Source: CAD feature listing. Evaluate the final solid. Frame: model axes, mm. A direction names the side the tool comes from. Coordinates: 2 decimals unless noted, no trailing zeros. Order: outer loops, then holes, each group sorted by start corner. A loop starts at its lowest first (then second) coordinate and runs counter-clockwise, first axis right, second up. Notation, with made-up numbers: (4.25, 51.25) -> (13.25, 51.25) arc R29 ccw to (13.25, 86.25) -> close; hole circle Ø3 at (15, -36.5). An arc over 180 degrees is marked (long way). Write item = value, one per line. Start each with the question number.
Item 1: Section query B-B (x = -144). Output: boundary loops of the cut face in (y, z).
Item 2: Ray query, line 1 along Z through (x, y) = (-213, -80); line 2 along X through (y, z) = (55, 34); line 3 along Y through (x, z) = (-111, 0). Return the intervals inside material, ascending. Write a range as [from, to].
Item 3: Mould query, pull axis X, two halves, no side actions, for faces 1 (the cylindrical face through (-129.529, -15.77, -50.076)), 2 (the flat face through (-95, -28, 0)), 3 (the cylindrical face through (-215.14, -80.33, -72.507)), 4 (the flat face through (-77.5, 22.3, -12.1)). Classes: released by +X, released by -X, zero draft, split by the parting line, or undercut.
Item 4: Set-up query: faces 5 (the flat face through (-215, -1, -105)), 6 (the cylindrical face through (-215.14, 75.436, 74.048)), 7 (the flat face through (-215, 105, -1)), 8 (the cylindrical face through (-9.86, 93.676, 1.139)), 9 (the flat face through (-205, 48, -48)). Return all of +Z, -Z, +X, -X, +Y, -Y with unobstructed straight access to the full face (end or side cutting, diameter ignored); none if empty.
Item 5: Section query D-D (y = -65.5). Output: boundary loops of the cut face in (x, z), then the cut area to 3 significant figures.
Item 6: Section query A-A (y = 97.5). Output: boundary loops of the cut face in (x, z), then the cut area to 3 significant figures.
Item 7: Section query C-C (z = 0). Count the separate pieces of the cut face and the enclosed holes in it, then the cut area to 3 significant figures.
Item 8: Contact query for flat-ended pins moving along their axis: pin 1 (6 mm diameter, centred on x = -219, y = 38, fed in from -Z); pin 2 (5 mm diameter, centred on x = -149, y = 18.5, fed in from +Z); pin 3 (6 mm diameter, centred on x = -114, y = 49.5, fed in from -Z); pin 4 (5 mm diameter, centred on x = -200.5, y = -76.5, fed in from +Z). Output: stop coordinate, or through.
```python
from build123d import *

# Parameters (mm, degrees)
CUT_EXTRUDE_1_REACH      = 275.542
SKETCH_2_R               = 8.75
PATTERN_CIRCULAR_1_COUNT = 4
SKETCH_3_W               = 210
SKETCH_3_H               = 210
SKETCH_3_R               = 28.7125
EXTRUDE_1_DEPTH          = 20
SKETCH_4_R               = 7.5
CUT_EXTRUDE_2_DEPTH      = 20
FILLET_1_R               = 22
PATTERN_CIRCULAR_5_COUNT = 4
FILLET_2_R               = 3
SKETCH_5_R               = 28.7125
SKETCH_5_R_2             = 27.5
EXTRUDE_2_DEPTH          = 17.5
FILLET_3_R               = 3


with BuildPart() as part:
    # Эскиз1 → Повернуть1 (revolve)
    with BuildSketch(Plane.XY, mode=Mode.PRIVATE) as revolve_1_sk:
        Polygon((0, 37.5), (0, 110), (-20, 110), (-20, 60), (-55, 52.5), (-205, 52.5), (-205, 105), (-225, 105), (-225, 62.5), (-210, 62.5), (-210, 28.7125), (-160, 28.7125), (-160, 40), (-95, 40), (-95, 28.7125), (-77.5, 28.7125), (-77.5, 25), align=None)
    revolve(revolve_1_sk.sketch.rotate(Axis((0, 0, 0), (-1, 0, 0)), 90), axis=Axis((0, 0, 0), (-1, 0, 0)))

    # Эскиз2 → Вырез-Вытянуть1 (cut, up to next)
    with BuildSketch(Plane(origin=(0, 0, 0), x_dir=(0, 0, -1), z_dir=(1, 0, 0)), mode=Mode.PRIVATE) as cut_extrude_1_sk1:
        with Locations((0, 85)):
            Circle(SKETCH_2_R)
    cut_extrude_1_tool1 = extrude(cut_extrude_1_sk1.sketch, amount=-CUT_EXTRUDE_1_REACH, mode=Mode.PRIVATE) & part.part
    cut_extrude_1 = cut_extrude_1_tool1.solids().sort_by_distance((0, 85, 0))[0]
    add(cut_extrude_1, mode=Mode.SUBTRACT)

    # Круговой массив1: Вырез-Вытянуть1 ×4 about axis
    pattern_circular_1_axis = Axis((0, 0, 0), (1, 0, 0))
    for i in range(1, PATTERN_CIRCULAR_1_COUNT):
        add(cut_extrude_1.rotate(pattern_circular_1_axis, i * 360 / PATTERN_CIRCULAR_1_COUNT), mode=Mode.SUBTRACT)

    # Эскиз3 → Бобышка-Вытянуть1 (add)
    with BuildSketch(Plane.ZY.offset(225)):
        Rectangle(SKETCH_3_W, SKETCH_3_H)
        with Locations(Location((0, 0, 0), (0, 0, 180))):
            Circle(SKETCH_3_R, mode=Mode.SUBTRACT)
    extrude(amount=-EXTRUDE_1_DEPTH)

    # Эскиз4 → Вырез-Вытянуть2 (cut)
    with BuildSketch(Plane.ZY.offset(225)):
        with Locations((80, 80)):
            Circle(SKETCH_4_R)
    cut_extrude_2 = extrude(amount=-CUT_EXTRUDE_2_DEPTH, mode=Mode.SUBTRACT)

    # Скругление1
    fillet_1_edges = [part.edges().sort_by_distance(p)[0] for p in [
        (-215, 105, 105),
        (-215, -105, 105),
        (-215, -105, -105),
        (-215, 105, -105),
    ]]
    fillet(fillet_1_edges, radius=FILLET_1_R)

    # Круговой массив5: Вырез-Вытянуть2 ×4 about axis
    pattern_circular_5_axis = Axis((0, 0, 0), (1, 0, 0))
    for i in range(1, PATTERN_CIRCULAR_5_COUNT):
        add(cut_extrude_2.rotate(pattern_circular_5_axis, i * 360 / PATTERN_CIRCULAR_5_COUNT), mode=Mode.SUBTRACT)

    # Скругление2
    fillet_2_edges = [part.edges().sort_by_distance(p)[0] for p in [
        (-160, 0, 40),
        (-95, 0, 40),
    ]]
    fillet(fillet_2_edges, radius=FILLET_2_R)

    # Эскиз5 → Бобышка-Вытянуть2 (add)
    with BuildSketch(Plane.ZY.offset(77.5)):
        with Locations(Location((0, 0, 0), (0, 0, 180))):
            Circle(SKETCH_5_R)
        with Locations(Location((0, 0, 0), (0, 0, 180))):
            Circle(SKETCH_5_R_2, mode=Mode.SUBTRACT)
    extrude(amount=EXTRUDE_2_DEPTH)

    # Скругление3
    fillet_3_edges = [part.edges().sort_by_distance(p)[0] for p in [
        (-20, 0, 60),
        (-205, 0, 52.5),
    ]]
    fillet(fillet_3_edges, radius=FILLET_3_R)


solid = part.part
```
Computed:
q1.outline = circle Ø105 at (0, 0); hole circle Ø80 at (0, 0)
q2.line_1 = [-105, -87.5], [-72.5, 72.5], [87.5, 105]
q2.line_2 = [-225, -205], [-20, 0]
q2.line_3 = [-52.5, -40], [40, 52.5]
q3.face_1 = undercut
q3.face_2 = undercut
q3.face_3 = zero draft
q3.face_4 = released by -X
q4.face_5 = -Z, -X, +Y, -Y
q4.face_6 = -X
q4.face_7 = +Z, -Z, -X, +Y
q4.face_8 = +X
q4.face_9 = none
q5.outline = (-225, -105) -> (-205, -105) -> (-205, 105) -> (-225, 105) -> close; (-20, -88.37) -> (0, -88.37) -> (0, 88.37) -> (-20, 88.37) -> close
q5.area = 7,730 mm^2
q6.outline = (-225, -99.55) -> (-205, -99.55) -> (-205, 99.55) -> (-225, 99.55) -> close; (-20, -50.93) -> (0, -50.93) -> (0, 50.93) -> (-20, 50.93) -> close
q6.area = 6,020 mm^2
q7.separate_pieces = 4
q7.enclosed_holes = 0
q7.area = 12,900 mm^2
q8.pin_1 = -105
q8.pin_2 = 50
q8.pin_3 = -24.37
q8.pin_4 = through
